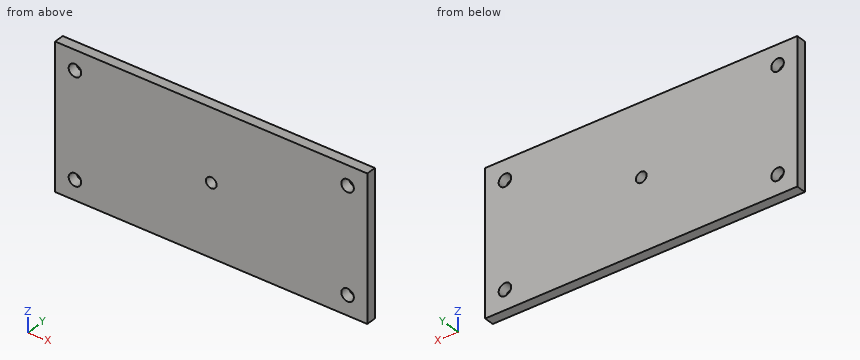
```python
from build123d import *

# Parameters (mm, degrees)
SKETCH1_W                   = 158
SKETCH1_H                   = 73
RIGHT_WALL_DEPTH            = 5
F_1_4_0_2500_DOWEL_HOLE1_D  = 6.35
TAP_DRILL_FOR_1_4_28_TAP2_D = 5.4102


with BuildPart() as part:
    # Sketch1 → right wall (new body)
    with BuildSketch(Plane(origin=(0, 0, 0), x_dir=(1, 0, 0), z_dir=(0, 1, 0))):
        with Locations((79, 36.5)):
            Rectangle(SKETCH1_W, SKETCH1_H)
    extrude(amount=RIGHT_WALL_DEPTH)

    # 1/4 (0.2500) Dowel Hole1 (through all)
    with Locations(Plane(origin=(0, 0, 0), x_dir=(-1, 0, 0), z_dir=(0, -1, 0))):
        with Locations((-10, 10), (-10, 63), (-148, 63), (-148, 10)):
            Hole(F_1_4_0_2500_DOWEL_HOLE1_D / 2)

    # Tap Drill for 1/4-28 Tap2 (through all)
    with Locations(Plane(origin=(0, 0, 0), x_dir=(-1, 0, 0), z_dir=(0, -1, 0))):
        with Locations((-79, 36.5)):
            Hole(TAP_DRILL_FOR_1_4_28_TAP2_D / 2)


solid = part.part
```
Design review of the part built by this model. Coordinates are the model's own, in mm. Round coordinates to 2 decimals unless told otherwise and drop trailing zeros. Order: outer loops, then holes, each group sorted by start corner. A loop starts at its lowest first (then second) coordinate and runs counter-clockwise, first axis right, second up. Notation, with made-up numbers: M 82.5,-23 L 132.5,-23 A24 cw 132.5,-9 Z; hole C -20.5,-31.75 d11. An arc over 180 degrees is marked long. Put each result on its own line as item: value.
Q1. Consider section C-C (z = -63). State the section outline as (x, y) points (3 decimals), and give its area (4 significant figures).
Reported:
outline: M 0,0 L 6.825,0 L 6.825,5 L 0,5 Z; M 13.175,0 L 144.825,0 L 144.825,5 L 13.175,5 Z; M 151.175,0 L 158,0 L 158,5 L 151.175,5 Z
area: 726.5 mm²
Q2. Consider section A-A (x = 148). State the section outline as (y, z) points (3 decimals), and give its area (4 significant figures).
Reported:
outline: M 0,-73 L 5,-73 L 5,-66.175 L 0,-66.175 Z; M 0,-59.825 L 5,-59.825 L 5,-13.175 L 0,-13.175 Z; M 0,-6.825 L 5,-6.825 L 5,0 L 0,0 Z
area: 301.5 mm²
Q3. To check wall thickness, follow line 1 (X direction, y = 2.95, z = -63) (3 decimals); line 2 (Z direction, x = 10, y = 1.5) (3 decimals); line 3 (X direction, y = 1, z = -36.5). State the ranges of each line that lie inside material, in increasing order.
Reported:
line 1: 0 to 6.825, 13.175 to 144.825, 151.175 to 158
line 2: -73 to -66.175, -59.825 to -13.175, -6.825 to 0
line 3: 0 to 76.29, 81.71 to 158
Q4. Consider section B-B (x = 79). State the section outline as (y, z) points.
Reported:
outline: M 0,-73 L 5,-73 L 5,-39.21 L 0,-39.21 Z; M 0,-33.79 L 5,-33.79 L 5,0 L 0,0 Z
Q5. Insertion check: pin 1 Ø5 at (x, z) = (10, -10) entering from -Y. The pin has a flat end and moves straight along its axis. Give the tip position at first contact, or say it passes through.
Reported:
pin 1: through
